Source: three-view drawing plus pictorial views. Frame: mm from the lowest corner of the part. Coordinates: 2 decimals unless noted, no trailing zeros. Write each loop counter-clockwise with the first axis right and the second up, starting at its lowest first coordinate (ties: lowest second). Pieces come first, ordered by that corner, then holes. Notation, with made-up numbers: (-37.75, 81) - (-0.75, 81) arc R15 cw to (-0.75, 90) - close; hole circle Ø8 at (57.5, 29.25). An arc over 180 degrees is marked (long way). Answer as a JSON object with one key per item and string values. Group by question number.
Item 1: Section A-A on z = 45. Return loops of the section in (x, y).
Item 2: Line query: line 1 along X through (y, z) = (76.5, 10); line 2 along Z through (x, y) = (90, 60); line 3 along X through (y, z) = (48, 50.5). Output: solid intervals per line, ascending. Write a range as from..to.
Item 3: First-contact query: pin 1 Ø6 at (x, z) = (10, 10) entering from -Y. Flat tip, straight axial feed; report the tip coordinate or a pass-through.
Item 4: Mould query, pull axis Z, two halves, no side actions, for the marked faces 1, 2 and 3. Classes: pulls with the +Z half, pulls with the -Z half, needs draft (parallel to the pull), parting line crosses it, or undercut.
Item 5: Section B-B on x = 50. Return loops of the section in (y, z), and give its area (3 significant figures).
Item 6: Section C-C on y = 19.5. Return loops of the section in (x, z), and give its area (3 significant figures).
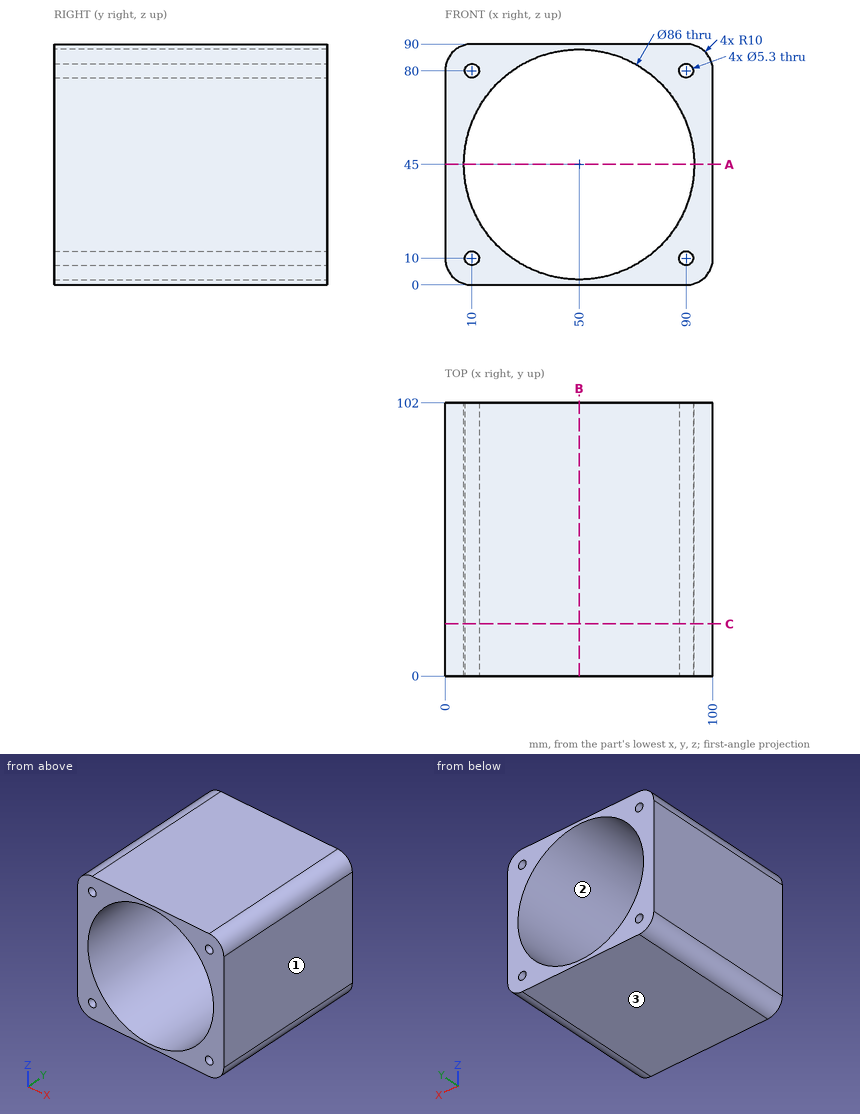
Checks:
{
 "1": {"outline": "(0, 0) - (7, 0) - (7, 102) - (0, 102) - close; (93, 0) - (100, 0) - (100, 102) - (93, 102) - close"},
 "2": {"line 1": "0..7.35, 12.65..25.02, 74.98..87.35, 92.65..100", "line 2": "0..7.35, 12.65..29.22, 60.78..77.35, 82.65..90", "line 3": "0..7.35, 92.65..100"},
 "3": {"pin 1": "y = 0"},
 "4": {"face 1": "needs draft", "face 2": "undercut", "face 3": "pulls with the -Z half"},
 "5": {"outline": "(0, 0) - (102, 0) - (102, 2) - (0, 2) - close; (0, 88) - (102, 88) - (102, 90) - (0, 90) - close", "area": "408 mm^2"},
 "6": {"outline": "(0, 10) arc R10 ccw to (10, 0) - (90, 0) arc R10 ccw to (100, 10) - (100, 80) arc R10 ccw to (90, 90) - (10, 90) arc R10 ccw to (0, 80) - close; hole circle Ø86 at (50, 45); hole circle Ø5.3 at (10, 10); hole circle Ø5.3 at (10, 80); hole circle Ø5.3 at (90, 10); hole circle Ø5.3 at (90, 80)", "area": "3,020 mm^2"}
}
